```python
from build123d import *

# Parameters (mm, degrees)
SKETCH_1_R          = 3
EXTRUDE_1_DEPTH     = 16
SKETCH_3_W          = 16
SKETCH_3_H          = 32
EXTRUDE_2_DEPTH     = 36
SKETCH_5_R          = 3
CUT_EXTRUDE_1_DEPTH = 36
SKETCH_8_R          = 18
CUT_EXTRUDE_6_DEPTH = 8


with BuildPart() as part:
    # 草图1 → 凸台-拉伸1 (new body)
    with BuildSketch(Plane(origin=(0, 0, 0), x_dir=(0, 0, -1), z_dir=(1, 0, 0))):
        with BuildLine():
            Line((-18, 0), (-18, 80))
            Line((-18, 80), (18, 80))
            Line((18, 80), (18, 0))
            ThreePointArc((18, 0), (0, -18), (-18, 0))
        make_face()
        Circle(SKETCH_1_R, mode=Mode.SUBTRACT)
    extrude(amount=EXTRUDE_1_DEPTH)

    # 草图3 → 凸台-拉伸2 (add)
    with BuildSketch(Plane(origin=(0, 0, -18), x_dir=(-1, 0, 0), z_dir=(0, 0, -1))):
        with Locations((-24, 64)):
            Rectangle(SKETCH_3_W, SKETCH_3_H)
    extrude(amount=-EXTRUDE_2_DEPTH)

    # 草图5 → 切除-拉伸1 (cut)
    with BuildSketch(Plane(origin=(0, 0, -18), x_dir=(-1, 0, 0), z_dir=(0, 0, -1))):
        with Locations((-16, 64)):
            Circle(SKETCH_5_R)
        with BuildLine():
            Line((-16, 92.996070946), (8.992787367, 92.996070946))
            Line((8.992787367, 92.996070946), (8.992787367, 64))
            Line((8.992787367, 64), (0, 64))
            ThreePointArc((0, 64), (-27.313708499, 75.313708499), (-16, 48))
            Line((-16, 48), (-16, 39.001100245))
            Line((-16, 39.001100245), (-49.117406919, 39.001100245))
            Line((-49.117406919, 39.001100245), (-49.117406919, 92.996070946))
            Line((-49.117406919, 92.996070946), (-16, 92.996070946))
        make_face()
    extrude(amount=-CUT_EXTRUDE_1_DEPTH, mode=Mode.SUBTRACT)

    # 草图8 → 切除-拉伸6 (cut, symmetric)
    with BuildSketch(Plane.XY):
        with Locations((16, 64)):
            Circle(SKETCH_8_R)
    extrude(amount=CUT_EXTRUDE_6_DEPTH, both=True, mode=Mode.SUBTRACT)


solid = part.part
```
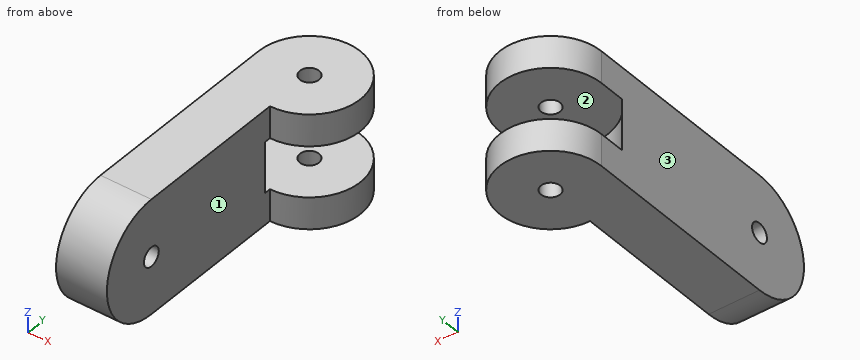
Geometry check sheet. Reference: the model listing, model coordinates, mm. Face numbers are marked on the shaded views. A direction names the side the tool comes from. Coordinates: 2 decimals unless noted, no trailing zeros. Loops run counter-clockwise (first coordinate to the right, second up) from the corner with the lowest first, then second, coordinate; pieces in that order, holes last.
Item 1: Sectioned sample at B-B, the plane x = 22.5. Record the boundary of the cut face in (y, z), then the cut area to 3 significant figures.
Item 2: Go/stop test with flat-tipped pins: pin 1 Ø8 at (y, z) = (0, 0) entering from +X; pin 2 Ø6 at (x, z) = (21, -14) entering from -Y; pin 3 Ø5.5 at (x, y) = (16, 64) entering from +Z. Record where each tip stops, or that it passes through.
Item 3: Sectioned sample at A-A, the plane z = 0. Record the boundary of the cut face in (x, y), then the cut area to 3 significant figures.
Item 4: Thickness scan on line 1 (Z direction, x = 8.5, y = 51); line 2 (X direction, y = 15, z = 14); line 3 (Y direction, x = 11.5, z = 0). Record the ranges inside material, lowest first.
Item 5: Sectioned sample at D-D, the plane y = 43.5. Record the boundary of the cut face in (x, z), then the cut area to 3 significant figures.
Item 6: Access from +Z, -Z, +X, -X, +Y, -Y to the whole of each face (thin tool, end or side, straight path). Record for the marked faces 1, 2 and 3.
Item 7: Sectioned sample at C-C, the plane z = -10.5. Record the boundary of the cut face in (x, y).
Check result:
1. outline: (49.38, -18) - (78.62, -18) - (78.62, -8) - (49.38, -8) - close; (49.38, 8) - (78.62, 8) - (78.62, 18) - (49.38, 18) - close
1. area: 585 mm2
2. pin 1: stops at x = 16
2. pin 2: stops at y = 48.13
2. pin 3: passes through
3. outline: (0, -18) - (16, -18) - (16, -3) - (0, -3) - close; (0, 3) - (16, 3) - (16, 46) arc R18 cw to (0, 55.75) - close
3. area: 973 mm2
4. line 1: z = -18 to -8, 8 to 18
4. line 2: x = 0 to 16
4. line 3: y = -18 to -3, 3 to 46.57
5. outline: (0, -18) - (16, -18) - (16, 18) - (0, 18) - close
5. area: 576 mm2
6. face 1: +Z, -Z, +X, -Y
6. face 2: +X, +Y
6. face 3: +Z, -Z, -X, +Y, -Y
7. outline: (0, -14.62) - (16, -14.62) - (16, 48) arc R16 ccw (long way) to (0, 64) - close; hole circle Ø6 at (16, 64)
